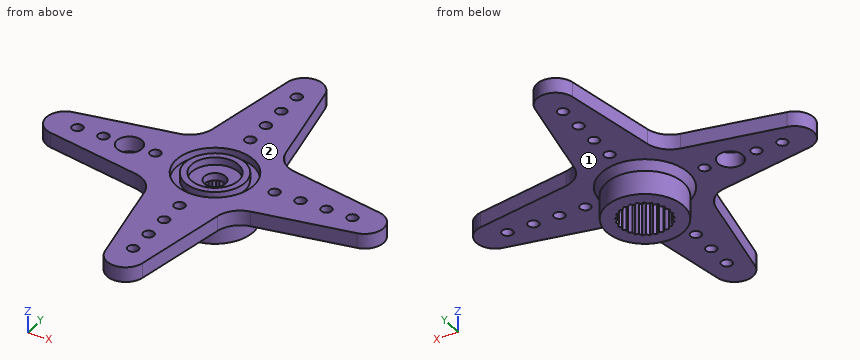
```python
from build123d import *

# Parameters (mm, degrees)
SKETCH1_R           = 4.5000037
BOSS_EXTRUDE1_DEPTH = 3.75000012
BOSS_EXTRUDE2_START = 1.750000056
SKETCH2_R           = 4.5000037
SKETCH2_R_2         = 3.499999998
SKETCH2_R_3         = 1.25000004
BOSS_EXTRUDE2_DEPTH = 1.750000056
SKETCH4_R           = 2.75000466
SKETCH4_R_2         = 1.25000004
CUT_EXTRUDE1_DEPTH  = 0.875000028
SKETCH6_R           = 4.5000037
SKETCH6_R_2         = 3.5000057
CUT_EXTRUDE2_DEPTH  = 0.875000028
SKETCH10_R          = 0.62500002
SKETCH10_R_2        = 4.5000037
BOSS_EXTRUDE4_DEPTH = 1.750000056
CHAMFER2_SIZE       = 1.00000054
CHAMFER2_SIZE2      = 0.577350581
SKETCH32_R          = 1.4605
CUT_EXTRUDE8_DEPTH  = 36.768264294


with BuildPart() as part:
    # Sketch1 → Boss-Extrude1 (new body)
    with BuildSketch(Plane.XY):
        with Locations((-10.24995918, 0)):
            Circle(SKETCH1_R)
        Polygon((-10.24995918, 2.999994), (-10.594624819, 2.728309468), (-10.996027349, 2.905743672), (-11.262299488, 2.55687975), (-11.695217312, 2.628914782), (-11.866365092, 2.224791874), (-12.303596391, 2.186901508), (-12.368865968, 1.752912142), (-12.782937891, 1.60747717), (-12.738228138, 1.170890494), (-13.103123023, 0.927049129), (-12.951243218, 0.515297489), (-13.244033377, 0.188371182), (-12.994526687, -0.172673551), (-13.196815038, -0.562142819), (-12.865358886, -0.849794878), (-12.964434908, -1.27733532), (-12.571855902, -1.473520467), (-12.561494285, -1.912268145), (-12.132459609, -2.004659346), (-12.01331141, -2.427046129), (-11.574778889, -2.409838105), (-11.354330629, -2.789323879), (-10.933854876, -2.663597874), (-10.625958129, -2.976338151), (-10.24995918, -2.749993992), (-9.873960231, -2.976338151), (-9.566063484, -2.663597874), (-9.145587731, -2.789323879), (-8.925139471, -2.409838105), (-8.48660695, -2.427046129), (-8.367458751, -2.004659346), (-7.938424075, -1.912268145), (-7.928062458, -1.473520467), (-7.535483452, -1.27733532), (-7.634559474, -0.849794878), (-7.303103322, -0.562142819), (-7.505391673, -0.172673551), (-7.255884983, 0.188371182), (-7.548675142, 0.515297489), (-7.396795337, 0.927049129), (-7.761690222, 1.170890494), (-7.716980469, 1.60747717), (-8.131052392, 1.752912142), (-8.196321969, 2.186901508), (-8.633553268, 2.224791874), (-8.804701048, 2.628914782), (-9.237618872, 2.55687975), (-9.503891011, 2.905743672), (-9.905293541, 2.728309468), align=None, mode=Mode.SUBTRACT)
    extrude(amount=-BOSS_EXTRUDE1_DEPTH)

    # Sketch2 → Boss-Extrude2 (add)
    # profile 1 of 2: a face of its own
    with BuildSketch(Plane.XY.offset(BOSS_EXTRUDE2_START)):
        with Locations((-10.24995918, 0)):
            Circle(SKETCH2_R)
        with Locations((-10.24995918, 0)):
            Circle(SKETCH2_R_2, mode=Mode.SUBTRACT)
    # profile 2 of 2: a face of its own
    with BuildSketch(Plane.XY.offset(BOSS_EXTRUDE2_START)):
        with Locations((-10.24995918, 0)):
            Circle(SKETCH2_R_2)
        with Locations((-10.24995918, 0)):
            Circle(SKETCH2_R_3, mode=Mode.SUBTRACT)
    extrude(amount=-BOSS_EXTRUDE2_DEPTH)

    # Sketch4 → Cut-Extrude1 (cut)
    with BuildSketch(Plane.XY.offset(1.750000056)):
        with Locations((-10.24995918, 0)):
            Circle(SKETCH4_R)
        with Locations((-10.24995918, 0)):
            Circle(SKETCH4_R_2, mode=Mode.SUBTRACT)
    extrude(amount=-CUT_EXTRUDE1_DEPTH, mode=Mode.SUBTRACT)

    # Sketch6 → Cut-Extrude2 (cut)
    with BuildSketch(Plane.XY.offset(1.750000056)):
        with Locations((-10.24995918, 0)):
            Circle(SKETCH6_R)
        with Locations((-10.24995918, 0)):
            Circle(SKETCH6_R_2, mode=Mode.SUBTRACT)
    extrude(amount=-CUT_EXTRUDE2_DEPTH, mode=Mode.SUBTRACT)

    # Sketch10 → Boss-Extrude4 (add)
    with BuildSketch(Plane.XY.offset(1.750000056)):
        with BuildLine():
            Line((-8.086927824, 17.701557226), (-6.029886341, 6.622035833))
            ThreePointArc((-6.029886341, 6.622035833), (-5.20161423, 5.04834495), (-3.627923347, 4.220072839))
            Line((-3.627923347, 4.220072839), (7.451598046, 2.163031356))
            ThreePointArc((7.451598046, 2.163031356), (9.25000182, 0), (7.451598046, -2.163031356))
            Line((7.451598046, -2.163031356), (-3.627923347, -4.220072839))
            ThreePointArc((-3.627923347, -4.220072839), (-5.20161423, -5.04834495), (-6.029886341, -6.622035833))
            Line((-6.029886341, -6.622035833), (-8.086927824, -17.701557226))
            ThreePointArc((-8.086927824, -17.701557226), (-10.24995918, -19.499961), (-12.412990536, -17.701557226))
            Line((-12.412990536, -17.701557226), (-14.470032019, -6.622035833))
            ThreePointArc((-14.470032019, -6.622035833), (-15.29830413, -5.04834495), (-16.871995013, -4.220072839))
            Line((-16.871995013, -4.220072839), (-27.951516406, -2.163031356))
            ThreePointArc((-27.951516406, -2.163031356), (-29.74992018, 0), (-27.951516406, 2.163031356))
            Line((-27.951516406, 2.163031356), (-16.871995013, 4.220072839))
            ThreePointArc((-16.871995013, 4.220072839), (-15.29830413, 5.04834495), (-14.470032019, 6.622035833))
            Line((-14.470032019, 6.622035833), (-12.412990536, 17.701557226))
            ThreePointArc((-12.412990536, 17.701557226), (-10.24995918, 19.499961), (-8.086927824, 17.701557226))
        make_face()
        with Locations((-10.24995918, 15.87496698)):
            Circle(SKETCH10_R, mode=Mode.SUBTRACT)
        with Locations((-10.24995918, 12.87497298)):
            Circle(SKETCH10_R, mode=Mode.SUBTRACT)
        with Locations((-10.24995918, 9.87497898)):
            Circle(SKETCH10_R, mode=Mode.SUBTRACT)
        with Locations((-10.24995918, 6.87498498)):
            Circle(SKETCH10_R, mode=Mode.SUBTRACT)
        with Locations((5.6250078, 0)):
            Circle(SKETCH10_R, mode=Mode.SUBTRACT)
        with Locations((2.6250138, 0)):
            Circle(SKETCH10_R, mode=Mode.SUBTRACT)
        with Locations((-0.3749802, 0)):
            Circle(SKETCH10_R, mode=Mode.SUBTRACT)
        with Locations((-3.3749742, 0)):
            Circle(SKETCH10_R, mode=Mode.SUBTRACT)
        with Locations((-10.24995918, -15.87496698)):
            Circle(SKETCH10_R, mode=Mode.SUBTRACT)
        with Locations((-10.24995918, -12.87497298)):
            Circle(SKETCH10_R, mode=Mode.SUBTRACT)
        with Locations((-10.24995918, -9.87497898)):
            Circle(SKETCH10_R, mode=Mode.SUBTRACT)
        with Locations((-10.24995918, -6.87498498)):
            Circle(SKETCH10_R, mode=Mode.SUBTRACT)
        with Locations((-26.12492616, 0)):
            Circle(SKETCH10_R, mode=Mode.SUBTRACT)
        with Locations((-23.12493216, 0)):
            Circle(SKETCH10_R, mode=Mode.SUBTRACT)
        with Locations((-20.12493816, 0)):
            Circle(SKETCH10_R, mode=Mode.SUBTRACT)
        with Locations((-17.12494416, 0)):
            Circle(SKETCH10_R, mode=Mode.SUBTRACT)
        with Locations((-10.24995918, 0)):
            Circle(SKETCH10_R_2, mode=Mode.SUBTRACT)
    extrude(amount=-BOSS_EXTRUDE4_DEPTH)

    # Chamfer2
    chamfer2_edges = [part.edges().sort_by_distance(p)[0] for p in [
        (-14.74996288, 0, 0),
    ]]
    chamfer2_side = [part.faces().sort_by_distance(p)[0] for p in [
        (-14.74996288, 0, -1.87500006),
    ]]
    chamfer(chamfer2_edges, length=CHAMFER2_SIZE, length2=CHAMFER2_SIZE2, reference=chamfer2_side[0])

    # Sketch32 → Cut-Extrude8 (cut, through all)
    with BuildSketch(Plane(origin=(0, 0, 0), x_dir=(-1, 0, 0), z_dir=(0, 0, -1))):
        with Locations((20.12493816, 0)):
            Circle(SKETCH32_R)
    extrude(amount=-CUT_EXTRUDE8_DEPTH, mode=Mode.SUBTRACT)


solid = part.part
```
The listing builds one solid part. Answer for the finished solid, in the listing's coordinates (mm). Face numbers are marked on the shaded views. A direction names the side the tool comes from. Give positions to 0.01 mm unless a question says otherwise; leave off trailing zeros. Write each loop counter-clockwise with the first axis right and the second up, starting at its lowest first coordinate (ties: lowest second). Pieces come first, ordered by that corner, then holes. Notation, with made-up numbers: (5.25, 55.5) -> (61.25, 55.5) arc R18 ccw to (61.25, 68.5) -> close; hole circle Ø8 at (3, 70). An arc over 180 degrees is marked (long way). Write item = value, one per line. Start each with the question number.
1) The part is cut by section A-A, the plane x = 2.5. Determine the outline of the cut face in (y, z).
2) Each of these flat-tipped pins is pushed along its axis until it touches: pin 1 (2 mm diameter, centred on x = -7, z = -1.5, fed in from -Y); pin 2 (2 mm diameter, centred on x = -10.25, y = -9.87, fed in from +Z); pin 3 (1.8 mm diameter, centred on x = -9.5, y = 1, fed in from -Z); pin 4 (2 mm diameter, centred on x = -21, z = 0, fed in from -Y). Where does it stop, or does it pass through?
3) Which of the six approach directions +Z, -Z, +X, -X, +Y, -Y give full straight-line access (tool end or side, diameter ignored) to the marked faces 1 and 2?
4) The part is cut by section B-B, the plane y = 14. Determine the outline of the cut face in (x, z), and give its area (3 significant figures).
5) Straight lines are drawn through the part: line 1 along Z through (x, y) = (-25, -2); line 2 along Y through (x, z) = (2.5, 0.1); line 3 along X through (y, z) = (-14, 0.45). For each, find the intervals that lie inside material, in ascending order.
Solutions:
q1.outline = (-3.08, 0) -> (-0.61, 0) -> (-0.61, 1.75) -> (-3.08, 1.75) -> close; (0.61, 0) -> (3.08, 0) -> (3.08, 1.75) -> (0.61, 1.75) -> close
q2.pin_1 = -3.9
q2.pin_2 = 1.75
q2.pin_3 = 0
q2.pin_4 = -3.64
q3.face_1 = -Z
q3.face_2 = +Z, +X, -X, +Y, -Y
q4.outline = (-13.1, 0) -> (-7.4, 0) -> (-7.4, 1.75) -> (-13.1, 1.75) -> close
q4.area = 9.98 mm²
q5.line_1 = 0 to 1.75
q5.line_2 = -3.08 to -0.61, 0.61 to 3.08
q5.line_3 = -13.1 to -7.4
